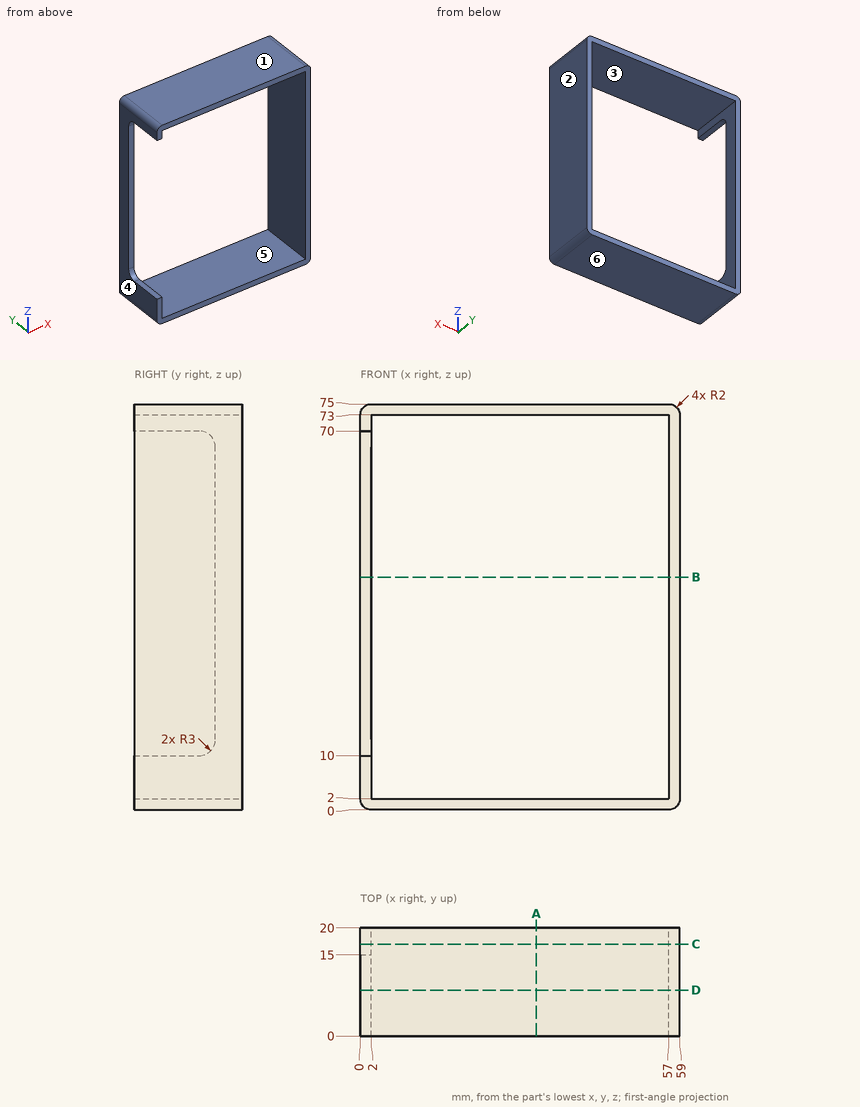
Could you check a few things on this drawing? It's one solid part, dimensions in mm from its lowest x, y, z. A direction names the side the tool comes from. Coordinates: 2 decimals unless noted, no trailing zeros. Write each loop counter-clockwise with the first axis right and the second up, starting at its lowest first coordinate (ties: lowest second). Pieces come first, ordered by that corner, then holes. Notation, with made-up numbers: (44, 36.25) - (49, 36.25) arc R34 cw to (49, 70.25) - close; hole circle Ø1 at (13.5, -19.5). An arc over 180 degrees is marked (long way). Put each result on its own line as item: value. Start each with the question number.
Q1. I want a section at D-D on y = 8.5. Write out the boundary of the cut face in (x, z).
Q2. Please list where these lines run through material, in increasing order: L1, parallel to X at y = 17.25, z = 34; L2, parallel to Z at x = 55, y = 15; L3, parallel to X at y = 3.75, z = 59.
Q3. Which directions (+Z, -Z, +X, -X, +Y, -Y) give clear straight access to the entire face, cutting with the end or side of a thin tool? Please do the marked faces 5 and 6.
Q4. I'm going to push flat-ended pins straight in: P1, Ø10, axis at y = 6, z = 29.5, coming from the -X side; P2, Ø1, axis at x = 1.5, z = 49.5, coming from the -Y side; P3, Ø12, axis at x = 46, z = 11.5, coming from the -Y side. Where does each tip first touch, or does it pass through?
Q5. I want a section at A-A on x = 32.5. Write out the boundary of the cut face in (y, z).
Q6. I want a section at B-B on z = 43. Write out the boundary of the cut face in (x, y), plus the area to 3 significant figures.
Q7. I want a section at C-C on y = 17. Write out the boundary of the cut face in (x, z).
Q8. Thinking about a two-plate mould opening in X: for the marked faces 1, 2, 3 and 4, which applies, pulls with the +X half, pulls with the -X half, needs draft (parallel to the pull), parting line crosses it, or undercut?
Checks:
1. outline: (0, 2) arc R2 ccw to (2, 0) - (57, 0) arc R2 ccw to (59, 2) - (59, 73) arc R2 ccw to (57, 75) - (2, 75) arc R2 ccw to (0, 73) - (0, 70) - (2, 70) - (2, 73) - (57, 73) - (57, 2) - (2, 2) - (2, 10) - (0, 10) - close
2. L1: 0 to 2, 57 to 59
2. L2: 0 to 2, 73 to 75
2. L3: 57 to 59
3. face 5: +Y, -Y
3. face 6: -Z, +X, -X, +Y, -Y
4. P1: x = 57
4. P2: y = 15
4. P3: through
5. outline: (0, 0) - (20, 0) - (20, 2) - (0, 2) - close; (0, 73) - (20, 73) - (20, 75) - (0, 75) - close
6. outline: (0, 15) - (2, 15) - (2, 20) - (0, 20) - close; (57, 0) - (59, 0) - (59, 20) - (57, 20) - close
6. area: 50.0 mm²
7. outline: (0, 2) arc R2 ccw to (2, 0) - (57, 0) arc R2 ccw to (59, 2) - (59, 73) arc R2 ccw to (57, 75) - (2, 75) arc R2 ccw to (0, 73) - close; hole (2, 2) - (57, 2) - (57, 73) - (2, 73) - close
8. face 1: needs draft
8. face 2: pulls with the +X half
8. face 3: undercut
8. face 4: pulls with the -X half
